Check sheet for the modelled part. Datum: model origin and axes. Units: mm. Coordinates: 2 decimals unless noted, no trailing zeros. Loops run counter-clockwise (first coordinate to the right, second up) from the corner with the lowest first, then second, coordinate; pieces in that order, holes last. Notation, with made-up numbers: (25.5, 18) - (83.5, 18) arc R12 cw to (83.5, 32) - close; hole circle Ø1 at (-27.5, -8). An arc over 180 degrees is marked (long way). Use a Markdown table: item, result. Add a question column.
1) Go/stop test with a flat-tipped pin: P1, Ø3, axis at x = 33, z = 3.5, coming from the +Y side. Record where the tip stops, or that it passes through.
2) Sectioned sample at C-C, the plane x = 30.5. Enter the section's corners in (y, z), then the cut area to 3 significant figures.
3) Sectioned sample at B-B, the plane x = 19.5. Enter the section's corners in (y, z).
4) Thickness scan on line 1 (X direction, y = -20.5, z = 3); line 2 (Y direction, x = 18, z = 5.4) (3 decimals); line 3 (Y direction, x = 22, z = 3). Record the ranges inside material, lowest first.
5) Sectioned sample at A-A, the plane z = 3.05. Enter the section's corners in (x, y), then the cut area to 3 significant figures.
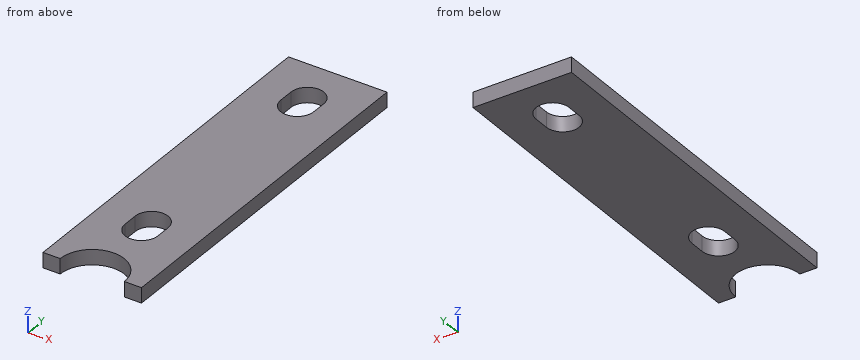
from build123d import *

# Parameters (mm, degrees)
SKETCH1_W           = 39
SKETCH1_H           = 145
BOSS_EXTRUDE1_DEPTH = 6
CUT_EXTRUDE2_DEPTH  = 6
CUT_EXTRUDE3_DEPTH  = 10


with BuildPart() as part:
    # Sketch1 → Boss-Extrude1 (new body)
    with BuildSketch(Plane.XY):
        with Locations((19.5, -72.5)):
            Rectangle(SKETCH1_W, SKETCH1_H)
    extrude(amount=BOSS_EXTRUDE1_DEPTH)

    # Sketch4 → Cut-Extrude2 (cut)
    with BuildSketch(Plane.XY.offset(6)):
        with BuildLine():
            Line((25.717260001, -109.5), (25.717260001, -115.5))
            ThreePointArc((25.717260001, -115.5), (19.217260001, -122), (12.717260001, -115.5))
            Line((12.717260001, -115.5), (12.717260001, -109.5))
            ThreePointArc((12.717260001, -109.5), (19.217260001, -103), (25.717260001, -109.5))
        make_face()
        with BuildLine():
            Line((25.717260001, -23.5), (25.717260001, -17.5))
            ThreePointArc((25.717260001, -17.5), (19.217260001, -11), (12.717260001, -17.5))
            Line((12.717260001, -17.5), (12.717260001, -23.5))
            ThreePointArc((12.717260001, -23.5), (19.217260001, -30), (25.717260001, -23.5))
        make_face()
    extrude(amount=-CUT_EXTRUDE2_DEPTH, mode=Mode.SUBTRACT)

    # Sketch5 → Cut-Extrude3 (cut)
    with BuildSketch(Plane.XY.offset(6)):
        with BuildLine():
            Line((6.8, -145), (32.2, -145))
            ThreePointArc((32.2, -145), (19.5, -132.3), (6.8, -145))
        make_face()
    extrude(amount=-CUT_EXTRUDE3_DEPTH, mode=Mode.SUBTRACT)


solid = part.part
Solved:
| question | item | result |
|---|---|---|
| 1 | P1 | stops at y = 0 |
| 2 | outline | (-138.65, 0) - (0, 0) - (0, 6) - (-138.65, 6) - close |
| 2 | area | 832 mm2 |
| 3 | outline | (-132.3, 0) - (-121.99, 0) - (-121.99, 6) - (-132.3, 6) - close; (-103.01, 0) - (-29.99, 0) - (-29.99, 6) - (-103.01, 6) - close; (-11.01, 0) - (0, 0) - (0, 6) - (-11.01, 6) - close |
| 4 | line 1 | x = 0 to 12.72, 25.72 to 39 |
| 4 | line 2 | y = -132.389 to -121.885, -103.115 to -29.885, -11.115 to 0 |
| 4 | line 3 | y = -132.55 to -121.37, -103.63 to -29.37, -11.63 to 0 |
| 5 | outline | (0, -145) - (6.8, -145) arc R12.7 cw to (32.2, -145) - (39, -145) - (39, 0) - (0, 0) - close; hole (12.72, -115.5) arc R6.5 ccw to (25.72, -115.5) - (25.72, -109.5) arc R6.5 ccw to (12.72, -109.5) - close; hole (12.72, -23.5) arc R6.5 ccw to (25.72, -23.5) - (25.72, -17.5) arc R6.5 ccw to (12.72, -17.5) - close |
| 5 | area | 4,980 mm2 |
